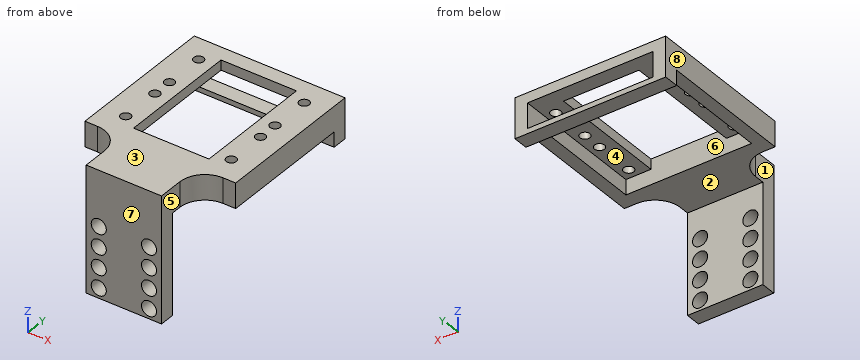
```python
from build123d import *

# Parameters (mm, degrees)
SKETCH1_W           = 30
SKETCH1_H           = 30
BOSS_EXTRUDE1_DEPTH = 5
SKETCH2_W           = 25
SKETCH2_H           = 24
CUT_EXTRUDE1_DEPTH  = 3
SKETCH3_W           = 15
SKETCH3_H           = 24
CUT_EXTRUDE2_DEPTH  = 22.424285286
SKETCH4_R           = 1
CUT_EXTRUDE3_DEPTH  = 22.424285286
SKETCH5_W           = 30
SKETCH5_H           = 3
BOSS_EXTRUDE2_DEPTH = 3
SKETCH6_R           = 1
CUT_EXTRUDE4_DEPTH  = 23.045407685
SKETCH7_W           = 25
SKETCH7_H           = 5
CUT_EXTRUDE5_DEPTH  = 4
SKETCH8_W           = 30
SKETCH8_H           = 3
CUT_EXTRUDE7_DEPTH  = 3
SKETCH9_W           = 30
SKETCH9_H           = 5
BOSS_EXTRUDE3_DEPTH = 10
SKETCH12_W          = 15
SKETCH12_H          = 3
BOSS_EXTRUDE5_DEPTH = 20
SKETCH13_W          = 7.5
SKETCH13_H          = 10
CUT_EXTRUDE9_DEPTH  = 36.355339059
SKETCH14_R          = 1.5
CUT_EXTRUDE10_DEPTH = 45.654227124
FILLET1_R           = 5
FILLET2_R           = 5


with BuildPart() as part:
    # Sketch1 → Boss-Extrude1 (new body)
    with BuildSketch(Plane.XY):
        Rectangle(SKETCH1_W, SKETCH1_H)
    extrude(amount=BOSS_EXTRUDE1_DEPTH)

    # Sketch2 → Cut-Extrude1 (cut)
    with BuildSketch(Plane(origin=(0, 0, 0), x_dir=(-1, 0, 0), z_dir=(0, 0, -1))):
        Rectangle(SKETCH2_W, SKETCH2_H)
    extrude(amount=-CUT_EXTRUDE1_DEPTH, mode=Mode.SUBTRACT)

    # Sketch3 → Cut-Extrude2 (cut, through all)
    with BuildSketch(Plane(origin=(0, 0, 3), x_dir=(-1, 0, 0), z_dir=(0, 0, -1))):
        Rectangle(SKETCH3_W, SKETCH3_H)
    extrude(amount=-CUT_EXTRUDE2_DEPTH, mode=Mode.SUBTRACT)

    # Sketch4 → Cut-Extrude3 (cut, through all)
    with BuildSketch(Plane(origin=(0, 0, 3), x_dir=(-1, 0, 0), z_dir=(0, 0, -1))):
        with Locations((10.5, 10)):
            Circle(SKETCH4_R)
        with Locations((10.5, -10)):
            Circle(SKETCH4_R)
        with Locations((-10.5, 10)):
            Circle(SKETCH4_R)
        with Locations((-10.5, -10)):
            Circle(SKETCH4_R)
    extrude(amount=-CUT_EXTRUDE3_DEPTH, mode=Mode.SUBTRACT)

    # Sketch5 → Boss-Extrude2 (add)
    with BuildSketch(Plane(origin=(0, 0, 0), x_dir=(-1, 0, 0), z_dir=(0, 0, -1))):
        with Locations((0, 13.5)):
            Rectangle(SKETCH5_W, SKETCH5_H)
        with Locations((0, -13.5)):
            Rectangle(SKETCH5_W, SKETCH5_H)
    extrude(amount=BOSS_EXTRUDE2_DEPTH)

    # Sketch6 → Cut-Extrude4 (cut, through all)
    with BuildSketch(Plane(origin=(0, 0, 3), x_dir=(-1, 0, 0), z_dir=(0, 0, -1))):
        with Locations((-10.5, 2)):
            Circle(SKETCH6_R)
        with Locations((-10.5, -2)):
            Circle(SKETCH6_R)
        with Locations((10.5, 2)):
            Circle(SKETCH6_R)
        with Locations((10.5, -2)):
            Circle(SKETCH6_R)
    extrude(amount=-CUT_EXTRUDE4_DEPTH, mode=Mode.SUBTRACT)

    # Sketch7 → Cut-Extrude5 (cut)
    with BuildSketch(Plane(origin=(0, 15, 0), x_dir=(1, 0, 0), z_dir=(0, 1, 0))):
        with Locations((0, -0.5)):
            Rectangle(SKETCH7_W, SKETCH7_H)
    extrude(amount=-CUT_EXTRUDE5_DEPTH, mode=Mode.SUBTRACT)

    # Sketch8 → Cut-Extrude7 (cut)
    with BuildSketch(Plane(origin=(0, 0, -3), x_dir=(-1, 0, 0), z_dir=(0, 0, -1))):
        with Locations((0, -13.5)):
            Rectangle(SKETCH8_W, SKETCH8_H)
    extrude(amount=-CUT_EXTRUDE7_DEPTH, mode=Mode.SUBTRACT)

    # Sketch9 → Boss-Extrude3 (add)
    with BuildSketch(Plane.XZ.offset(15)):
        with Locations((0, 2.5)):
            Rectangle(SKETCH9_W, SKETCH9_H)
    extrude(amount=BOSS_EXTRUDE3_DEPTH)

    # Sketch12 → Boss-Extrude5 (add)
    with BuildSketch(Plane(origin=(0, 0, 0), x_dir=(-1, 0, 0), z_dir=(0, 0, -1))):
        with Locations((0, -23.5)):
            Rectangle(SKETCH12_W, SKETCH12_H)
    extrude(amount=BOSS_EXTRUDE5_DEPTH)

    # Sketch13 → Cut-Extrude9 (cut, through all)
    with BuildSketch(Plane(origin=(0, 0, 0), x_dir=(-1, 0, 0), z_dir=(0, 0, -1))):
        with Locations((-11.25, -20)):
            Rectangle(SKETCH13_W, SKETCH13_H)
        with Locations((11.25, -20)):
            Rectangle(SKETCH13_W, SKETCH13_H)
    extrude(amount=-CUT_EXTRUDE9_DEPTH, mode=Mode.SUBTRACT)

    # Sketch14 → Cut-Extrude10 (cut, through all)
    with BuildSketch(Plane(origin=(0, -22, 0), x_dir=(1, 0, 0), z_dir=(0, 1, 0))):
        with Locations(Location((-5, 6, 0), (0, 0, 270))):
            Circle(SKETCH14_R)
        with Locations(Location((-5, 10, 0), (0, 0, 270))):
            Circle(SKETCH14_R)
        with Locations(Location((-5, 14, 0), (0, 0, 270))):
            Circle(SKETCH14_R)
        with Locations(Location((-5, 18, 0), (0, 0, 270))):
            Circle(SKETCH14_R)
        with Locations(Location((5, 6, 0), (0, 0, 270))):
            Circle(SKETCH14_R)
        with Locations(Location((5, 10, 0), (0, 0, 270))):
            Circle(SKETCH14_R)
        with Locations(Location((5, 14, 0), (0, 0, 270))):
            Circle(SKETCH14_R)
        with Locations(Location((5, 18, 0), (0, 0, 270))):
            Circle(SKETCH14_R)
    extrude(amount=-CUT_EXTRUDE10_DEPTH, mode=Mode.SUBTRACT)

    # Fillet1
    fillet1_edges = [part.edges().sort_by_distance(p)[0] for p in [
        (7.5, -15, 2.5),
    ]]
    fillet(fillet1_edges, radius=FILLET1_R)

    # Fillet2
    fillet2_edges = [part.edges().sort_by_distance(p)[0] for p in [
        (-7.5, -15, 2.5),
    ]]
    fillet(fillet2_edges, radius=FILLET2_R)


solid = part.part
```
Input: part model. Units: mm. Frame: model coordinates. Face numbers are marked on the shaded views. A direction names the side the tool comes from. Coordinates: 2 decimals unless noted, no trailing zeros. Loops run counter-clockwise (first coordinate to the right, second up) from the corner with the lowest first, then second, coordinate; pieces in that order, holes last.
Q1. Mould query, pull axis X, two halves, no side actions, for the marked faces 6, 7 and 8. Classes: +X half, -X half, draft (parallel to the pull), parting line (faces both ways), or undercut.
Results are:
face 6: undercut
face 7: draft
face 8: -X half
Q2. Line query: line 1 along X through (y, z) = (-23.65, -18); line 2 along X through (y, z) = (-4.5, 3.5); line 3 along Y through (x, z) = (-10.5, 4.25). Output: solid intervals per line, ascending.
Results are:
line 1: x = -7.5 to -6.5, -3.5 to 3.5, 6.5 to 7.5
line 2: x = -15 to -7.5, 7.5 to 15
line 3: y = -15.42 to -11, -9 to -3, -1 to 1, 3 to 9, 11 to 15
Q3. Section A-A, the plane x = -3. Return the cut outline in (y, z), and give its area (3 significant figures).
Results are:
outline: (-25, -20) - (-22, -20) - (-22, 0) - (-12, 0) - (-12, 5) - (-25, 5) - close; (12, -3) - (15, -3) - (15, -2) - (12, -2) - close; (12, 3) - (15, 3) - (15, 5) - (12, 5) - close
area: 134 mm2
Q4. Set-up query: the marked faces 1, 2, 3, 4 and 5. Return all of +Z, -Z, +X, -X, +Y, -Y with unobstructed straight access to the full face (end or side cutting, diameter ignored); none if empty.
Results are:
face 1: +Z, -Z, -X, -Y
face 2: -Z, +X, -X
face 3: +Z, +X, -X, +Y, -Y
face 4: +Y
face 5: +Z, -Z, +X, -Y
Q5. Section D-D, the plane x = 5. Give the number of separate pieces and of enclosed holes in the cut face, and give its area (3 significant figures).
Results are:
separate pieces: 7
enclosed holes: 0
area: 98.0 mm2
Q6. Contact query for flat-ended pins moving along their axis: pin 1 (3.5 mm diameter, centred on x = 5, z = -18, fed in from -Y); pin 2 (3.5 mm diameter, centred on x = -0.5, y = 13.5, fed in from -Z); pin 3 (1.6 mm diameter, centred on x = -10.5, y = 2, fed in from +Z); pin 4 (5.5 mm diameter, centred on y = -21.5, z = -2.5, fed in from -X). Output: stop coordinate, or through.
Results are:
pin 1: stops at y = -25
pin 2: stops at z = -3
pin 3: passes through
pin 4: stops at x = -7.5
Q7. Section B-B, the plane z = -10. Return the cut outline in (x, y).
Results are:
outline: (-7.5, -25) - (-6.5, -25) - (-6.5, -22) - (-7.5, -22) - close; (-3.5, -25) - (3.5, -25) - (3.5, -22) - (-3.5, -22) - close; (6.5, -25) - (7.5, -25) - (7.5, -22) - (6.5, -22) - close
Q8. Section C-C, the plane y = 0. Return the cut outline in (x, z).
Results are:
outline: (-15, 0) - (-12.5, 0) - (-12.5, 3) - (-7.5, 3) - (-7.5, 5) - (-15, 5) - close; (7.5, 3) - (12.5, 3) - (12.5, 0) - (15, 0) - (15, 5) - (7.5, 5) - close
